```python
from build123d import *

# Parameters (mm, degrees)
EXTRUDE_1_DEPTH     = 0.45
CUT_EXTRUDE_1_DEPTH = 5
SKETCH_6_R          = 0.5
SKETCH_6_R_2        = 0.75
CUT_EXTRUDE_4_DEPTH = 10.1
EXTRUDE_1_2_DEPTH   = 0.2
SKETCH_8_W          = 0.2
SKETCH_8_H          = 3.25
EXTRUDE_2_DEPTH     = 0.2
EXTRUDE_3_DEPTH     = 0.2


with BuildPart() as part:
    # Эскиз1 → Extrude 1 (new, symmetric)
    with BuildSketch(Plane.XY):
        with BuildLine():
            Line((-11.5, -18.5), (11.5, -18.5))
            Line((11.5, -18.5), (11.5, -6))
            ThreePointArc((11.5, -6), (9.732233047, -5.267766953), (9, -3.5))
            Line((9, -3.5), (5, -3.5))
            Line((5, -3.5), (5, -12))
            Line((5, -12), (-5, -12))
            Line((-5, -12), (-5, -3.5))
            Line((-5, -3.5), (-9, -3.5))
            Line((-9, -3.5), (-11.5, -3.5))
            Line((-11.5, -3.5), (-11.5, -6))
            Line((-11.5, -6), (-11.5, -18.5))
        make_face()
    extrude(amount=EXTRUDE_1_DEPTH, both=True)

    # Эскиз2 → Вырез-Вытянуть1 (cut, symmetric)
    with BuildSketch(Plane.XY):
        Polygon((-0.75, -15.25), (-0.75, -18.5), (0.75, -18.5), (0.75, -15.25), (0.75, -15.15), (-0.75, -15.15), align=None)
    extrude(amount=CUT_EXTRUDE_1_DEPTH, both=True, mode=Mode.SUBTRACT)

    # Эскиз6 → Вырез-Вытянуть4 (cut, symmetric)
    with BuildSketch(Plane.XY):
        with Locations((3.333333333, -13.5)):
            Circle(SKETCH_6_R)
        with Locations((-7.3, -8.75)):
            Circle(SKETCH_6_R)
        with Locations((-7.3, -5.5)):
            Circle(SKETCH_6_R)
        with Locations((7.3, -8.75)):
            Circle(SKETCH_6_R)
        with Locations((7.3, -5.5)):
            Circle(SKETCH_6_R)
        with Locations((-3.333333333, -13.5)):
            Circle(SKETCH_6_R)
        with Locations((-7.3, -12)):
            Circle(SKETCH_6_R)
        with Locations((7.3, -12)):
            Circle(SKETCH_6_R)
        with Locations((-9.5, -14.5)):
            Circle(SKETCH_6_R_2)
        with Locations((-9.3, -8.75)):
            Circle(SKETCH_6_R)
        with Locations((-9.3, -5.5)):
            Circle(SKETCH_6_R)
    extrude(amount=CUT_EXTRUDE_4_DEPTH, both=True, mode=Mode.SUBTRACT)

    # Эскиз7 → Extrude 1 2 (add)
    with BuildSketch(Plane.XY.offset(0.45)):
        Polygon((-7.335370626, -12.093535655), (-3.368703959, -13.593535655), (-3.297962707, -13.406464345), (-7.264629374, -11.906464345), align=None)
    extrude(amount=EXTRUDE_1_2_DEPTH)

    # Эскиз8 → Вытянуть-Тонкостенный2 (add)
    with BuildSketch(Plane(origin=(0, 0, -0.45), x_dir=(-1, 0, 0), z_dir=(0, 0, -1))):
        with Locations((9.4, -7.125)):
            Rectangle(SKETCH_8_W, SKETCH_8_H)
    extrude(amount=EXTRUDE_2_DEPTH)

    # Эскиз9 → Вытянуть-Тонкостенный3 (add)
    with BuildSketch(Plane.XY.offset(0.45)):
        Polygon((-9.3, -8.75), (-9.5, -14.5), (-9.699879127, -14.493047683), (-9.499879127, -8.743047683), align=None)
    extrude(amount=EXTRUDE_3_DEPTH)


solid = part.part
```
The listing builds one solid part. Answer for the finished solid, in the listing's coordinates (mm). A direction names the side the tool comes from. Give positions to 0.01 mm unless a question says otherwise; leave off trailing zeros. Order: outer loops, then holes, each group sorted by start corner. A loop starts at its lowest first (then second) coordinate and runs counter-clockwise, first axis right, second up. Notation, with made-up numbers: (-15.75, 81) -> (0.25, 81) arc R8 cw to (0.25, 94) -> close; hole circle Ø5 at (-33.75, -12.75). An arc over 180 degrees is marked (long way). One line per item, written item: value.
1) Find section B-B, the plane x = 7.3. Determine the outline of the cut face in (y, z).
Reported:
outline: (-18.5, -0.45) -> (-12.5, -0.45) -> (-12.5, 0.45) -> (-18.5, 0.45) -> close; (-11.5, -0.45) -> (-9.25, -0.45) -> (-9.25, 0.45) -> (-11.5, 0.45) -> close; (-8.25, -0.45) -> (-6, -0.45) -> (-6, 0.45) -> (-8.25, 0.45) -> close; (-5, -0.45) -> (-3.5, -0.45) -> (-3.5, 0.45) -> (-5, 0.45) -> close
2) A tool of negligible diameter and unlimited length cuts with its end or side. For faces 4 (the cylindrical face through (7.531, -9.194, 0.006)), 5 (the flat face through (-0.75, -17, 0)), 6 (the flat face through (-5, -8, 0)), from which of +Z, -Z, +X, -X, +Y, -Y can it reach the whole face along a straight path? Write none if from no direction.
Reported:
face 4: +Z, -Z
face 5: +Z, -Z, -Y
face 6: +Z, -Z, +Y
3) Find section A-A, the plane y = -16.75. Determine the outline of the cut face in (x, z), plus the area to 4 significant figures.
Reported:
outline: (-11.5, -0.45) -> (-0.75, -0.45) -> (-0.75, 0.45) -> (-11.5, 0.45) -> close; (0.75, -0.45) -> (11.5, -0.45) -> (11.5, 0.45) -> (0.75, 0.45) -> close
area: 19.35 mm^2
4) Determine the mould class of faces 1 (the flat face through (-6, -18.5, 0)), 2 (the cylindrical face through (9.752, -5.287, 0.006)), 3 (the cylindrical face through (-2.87, -13.69, 0.01)) for opening direction X: pulls with the +X half, pulls with the -X half, needs draft (parallel to the pull), parting line crosses it, or undercut.
Reported:
face 1: needs draft
face 2: pulls with the +X half
face 3: undercut
5) Find section D-D, the plane x = -0.25. Determine the outline of the cut face in (y, z).
Reported:
outline: (-15.15, -0.45) -> (-12, -0.45) -> (-12, 0.45) -> (-15.15, 0.45) -> close
6) Find the intervals of material crossed by line 1 (Y direction, x = -7.3, z = -0.1); line 2 (X direction, y = -13.5, z = 0.25); line 3 (X direction, y = -5.5, z = 0), in increasing order.
Reported:
line 1: y = -18.5 to -12.5, -11.5 to -9.25, -8.25 to -6, -5 to -3.5
line 2: x = -11.5 to -3.83, -2.83 to 2.83, 3.83 to 11.5
line 3: x = -11.5 to -9.8, -8.8 to -7.8, -6.8 to -5, 5 to 6.8, 7.8 to 10
7) Find section C-C, the plane z = -0.2. Count the separate pieces of the cut face and the enclosed holes in it, plus the area to 3 significant figures.
Reported:
separate pieces: 1
enclosed holes: 11
area: 240 mm^2
8) A flat-ended cylindrical pin translates along its axis: P1, Ø1.5, axis at x = -1, y = -14.5, coming from the +Z side. Find the tip coordinate at first contact, or state that the pin passes through.
Reported:
P1: stops at z = 0.45
